```python
from build123d import *

# Parameters (mm, degrees)
SKICA1_W                = 36
SKICA1_H                = 43
P_IDAT_VYSUNUT_M1_DEPTH = 3.5
P_IDAT_VYSUNUT_M2_DEPTH = 3
P_IDAT_VYSUNUT_M3_DEPTH = 3
ZAOBLIT1_R              = 2.5
ZAOBLIT2_R              = 0.5


with BuildPart() as part:
    # Skica1 → Přidat vysunutím1 (new body)
    with BuildSketch(Plane(origin=(0, 0, 0), x_dir=(0, 0, -1), z_dir=(1, 0, 0))):
        Rectangle(SKICA1_W, SKICA1_H)
    extrude(amount=P_IDAT_VYSUNUT_M1_DEPTH)

    # Skica2 → Přidat vysunutím2 (add)
    with BuildSketch(Plane(origin=(3.5, 0, 0), x_dir=(0, 0, -1), z_dir=(1, 0, 0))):
        with BuildLine():
            Line((-1.4, 15.48178046), (-1.4, -15.48178046))
            ThreePointArc((-1.4, -15.48178046), (0, -15.7), (1.4, -15.48178046))
            Line((1.4, -15.48178046), (1.4, 15.48178046))
            ThreePointArc((1.4, 15.48178046), (0, 15.7), (-1.4, 15.48178046))
        make_face()
    extrude(amount=P_IDAT_VYSUNUT_M2_DEPTH)

    # Skica3 → Přidat vysunutím3 (add)
    with BuildSketch(Plane(origin=(6.5, 0, 0), x_dir=(0, 0, -1), z_dir=(1, 0, 0))):
        with BuildLine():
            Line((-4.6, -11.1), (-4.6, 11.1))
            ThreePointArc((-4.6, 11.1), (0, 15.7), (4.6, 11.1))
            Line((4.6, 11.1), (4.6, -11.1))
            ThreePointArc((4.6, -11.1), (0, -15.7), (-4.6, -11.1))
        make_face()
    extrude(amount=P_IDAT_VYSUNUT_M3_DEPTH)

    # Zaoblit1
    zaoblit1_edges = [part.edges().sort_by_distance(p)[0] for p in [
        (1.75, -21.5, 18),
        (1.75, 21.5, 18),
    ]]
    fillet(zaoblit1_edges, radius=ZAOBLIT1_R)

    # Zaoblit2
    zaoblit2_edges = [part.edges().sort_by_distance(p)[0] for p in [
        (3.5, 0, -18),
        (0, -21.5, -1.25),
        (3.5, -21.5, -1.25),
        (0, 0, 18),
        (0, 20.767766953, 17.267766953),
        (0, -20.767766953, 17.267766953),
        (3.5, 0, 18),
        (3.5, 20.767766953, 17.267766953),
        (3.5, -20.767766953, 17.267766953),
        (0, 21.5, -1.25),
        (0, 0, -18),
        (3.5, 21.5, -1.25),
    ]]
    fillet(zaoblit2_edges, radius=ZAOBLIT2_R)


solid = part.part
```
Source: CAD feature listing. Evaluate the final solid. Frame: model axes, mm. A direction names the side the tool comes from. Give positions to 0.01 mm unless a question says otherwise; leave off trailing zeros. Order: outer loops, then holes, each group sorted by start corner. A loop starts at its lowest first (then second) coordinate and runs counter-clockwise, first axis right, second up.
(1) Section query C-C (y = -6). Return the cut outline in (x, z).
(2) Access query for faces 1 (the face through (8, 0, -4.6)), 2 (the face through (6.5, 0, 3)), 3 (the face through (8, 0, 4.6)), 4 (the face through (9.5, 0, 0)), 5 (the face through (5, 0, -1.4)). Directions: +Z, -Z, +X, -X, +Y, -Y. A direction counts if a zero-diameter tool reaches every point of the face in a straight line with its end or side. Return the directions, or none.
(3) Material intervals for line 1 along X through (y, z) = (9, -11.5); line 2 along X through (y, z) = (-11.5, -4.5); line 3 along Z through (x, y) = (7.25, 1), sorted ascending.
(4) Contact query for flat-ended pins moving along their axis: P1, Ø5, axis at x = 8, z = 5, coming from the +Y side; P2, Ø6, axis at y = -2, z = -11, coming from the +X side; P3, Ø0.9, axis at x = 4.5, y = -3.5, coming from the +Z side. Output: stop coordinate, or through.
(5) Section query B-B (z = 3). Return the cut outline in (x, y), plus the area to 3 significant figures.
(6) Section query D-D (x = 7.5). Return the cut outline in (y, z), plus the area to 3 significant figures.
(7) Pull-direction query (X, two-part tool) for faces 6 (the face through (2, 21, 17)), 7 (the face through (0, 0, 0)), 8 (the face through (6.5, 0, -3)); classes: +X half, -X half, draft (parallel to the pull), parting line (faces both ways), or undercut.
(8) Section query A-A (z = 7.5). Return the cut outline in (x, y).
Outcome:
1. outline: (0, -17.5) arc R0.5 ccw to (0.5, -18) - (3, -18) arc R0.5 ccw to (3.5, -17.5) - (3.5, -1.4) - (6.5, -1.4) - (6.5, -4.6) - (9.5, -4.6) - (9.5, 4.6) - (6.5, 4.6) - (6.5, 1.4) - (3.5, 1.4) - (3.5, 17.5) arc R0.5 ccw to (3, 18) - (0.5, 18) arc R0.5 ccw to (0, 17.5) - close
2. face 1: -Z, +X, +Y, -Y
2. face 2: +Z, +Y, -Y
2. face 3: +Z, +X, +Y, -Y
2. face 4: +Z, -Z, +X, +Y, -Y
2. face 5: -Z, +Y, -Y
3. line 1: x = 0 to 3.5
3. line 2: x = 0 to 3.5, 6.5 to 9.5
3. line 3: z = -4.6 to 4.6
4. P1: stops at y = 14.96
4. P2: stops at x = 3.5
4. P3: stops at z = 1.4
5. outline: (0, -21) arc R0.5 ccw to (0.5, -21.5) - (3, -21.5) arc R0.5 ccw to (3.5, -21) - (3.5, 21) arc R0.5 ccw to (3, 21.5) - (0.5, 21.5) arc R0.5 ccw to (0, 21) - close; (6.5, -14.59) - (9.5, -14.59) - (9.5, 14.59) - (6.5, 14.59) - close
5. area: 238 mm2
6. outline: (-11.1, -4.6) - (11.1, -4.6) arc R4.6 ccw to (11.1, 4.6) - (-11.1, 4.6) arc R4.6 ccw to start
6. area: 271 mm2
7. face 6: draft
7. face 7: -X half
7. face 8: undercut
8. outline: (0, -21) arc R0.5 ccw to (0.5, -21.5) - (3, -21.5) arc R0.5 ccw to (3.5, -21) - (3.5, 21) arc R0.5 ccw to (3, 21.5) - (0.5, 21.5) arc R0.5 ccw to (0, 21) - close
